Read the model definition and answer for the solid it produces. Units are mm, in the model's axes. A direction names the side the tool comes from. Give positions to 0.01 mm unless a question says otherwise; leave off trailing zeros. Write each loop counter-clockwise with the first axis right and the second up, starting at its lowest first coordinate (ties: lowest second). Pieces come first, ordered by that corner, then holes. Notation, with made-up numbers: (69.5, -26.75) -> (95.5, -26.75) arc R17 cw to (95.5, -10.75) -> close; hole circle Ø4 at (1.25, 78). An arc over 180 degrees is marked (long way). Use a Markdown table: item, result.
from build123d import *

# Parameters (mm, degrees)
SKETCH1_W           = 25.25
SKETCH1_H           = 12.5
BOSS_EXTRUDE1_DEPTH = 25.055
SKETCH2_W           = 14.5
SKETCH2_H           = 5.7
CUT_EXTRUDE1_DEPTH  = 10
BOSS_EXTRUDE2_DEPTH = 15.65
SKETCH4_R           = 4.715
BOSS_EXTRUDE3_DEPTH = 14.71
SKETCH5_R           = 2.875
SKETCH6_R           = 1.835
BOSS_EXTRUDE4_DEPTH = 10
SKETCH7_R           = 3
BOSS_EXTRUDE5_DEPTH = 5
SKETCH8_R           = 2.075
BOSS_EXTRUDE6_DEPTH = 10
FILLET1_R           = 3.67


with BuildPart() as part:
    # Sketch1 → Boss-Extrude1 (new, symmetric)
    with BuildSketch(Plane.XY):
        Rectangle(SKETCH1_W, SKETCH1_H)
    extrude(amount=BOSS_EXTRUDE1_DEPTH, both=True)

    # Sketch2 → Cut-Extrude1 (cut)
    with BuildSketch(Plane(origin=(0, 0, -25.055), x_dir=(-1, 0, 0), z_dir=(0, 0, -1))):
        with Locations((0, -1.17)):
            Rectangle(SKETCH2_W, SKETCH2_H)
    extrude(amount=-CUT_EXTRUDE1_DEPTH, mode=Mode.SUBTRACT)

    # Sketch3 → Boss-Extrude2 (add)
    with BuildSketch(Plane.XY.offset(25.055)):
        with BuildLine():
            Line((-6.42, 3.78), (-2.5, 3.78))
            ThreePointArc((-2.5, 3.78), (0.705, 0.575), (-2.5, -2.63))
            Line((-2.5, -2.63), (-6.42, -2.63))
            ThreePointArc((-6.42, -2.63), (-9.625, 0.575), (-6.42, 3.78))
        make_face()
    extrude(amount=BOSS_EXTRUDE2_DEPTH)

    # Sketch4 → Boss-Extrude3 (add)
    with BuildSketch(Plane.XY.offset(25.055)):
        with Locations(Location((5.61, -1.535, 0), (0, 0, 270))):
            Circle(SKETCH4_R)
    extrude(amount=BOSS_EXTRUDE3_DEPTH)

    # Sketch5 → section 1 of loft1
    with BuildSketch(Plane.XY.offset(59.725), mode=Mode.PRIVATE) as loft1_s1:
        with Locations((5.61, -1.535)):
            Circle(SKETCH5_R)
    # loft from a face of the part (loft1)
    loft([part.faces().sort_by_distance((5.61, -1.535, 39.765))[0], loft1_s1.sketch])

    # Sketch6 → Boss-Extrude4 (add)
    with BuildSketch(Plane.XY.offset(59.725)):
        with Locations((5.61, -1.535)):
            Circle(SKETCH6_R)
    extrude(amount=BOSS_EXTRUDE4_DEPTH)

    # Sketch7 → Boss-Extrude5 (add)
    with BuildSketch(Plane.XY.offset(40.705)):
        with Locations((-4.46, 0.575)):
            Circle(SKETCH7_R)
    extrude(amount=BOSS_EXTRUDE5_DEPTH)

    # Sketch8 → Boss-Extrude6 (add)
    with BuildSketch(Plane.XY.offset(45.705)):
        with Locations((-4.46, 0.575)):
            Circle(SKETCH8_R)
    extrude(amount=BOSS_EXTRUDE6_DEPTH)

    # Fillet1
    fillet1_edges = [part.edges().sort_by_distance(p)[0] for p in [
        (12.625, -6.25, 0),
        (-12.625, -6.25, 0),
        (-12.625, 6.25, 0),
        (12.625, 6.25, 0),
    ]]
    fillet(fillet1_edges, radius=FILLET1_R)


solid = part.part
Item 1: Straight lines are drawn through the part: line 1 along Z through (x, y) = (-8.5, -0.5) (3 decimals); line 2 along Z through (x, y) = (3.25, -0.5) (3 decimals); line 3 along Y through (x, z) = (5, 28.5). For each, find the intervals that lie inside material, in ascending order. Write a range as [from, to].
Return value:
| item | result |
|---|---|
| line 1 | [-25.055, 40.705] |
| line 2 | [-15.055, 59.725] |
| line 3 | [-6.21, 3.14] |
Item 2: A cutting plane is placed at A-A (x = -4.46). Give the vertices of the cut face in (y, z) (3 decimals), then the cut area to 3 significant figures.
Return value:
| item | result |
|---|---|
| outline | (-6.25, -25.055) -> (-4.02, -25.055) -> (-4.02, -15.055) -> (1.68, -15.055) -> (1.68, -25.055) -> (6.25, -25.055) -> (6.25, 25.055) -> (3.78, 25.055) -> (3.78, 40.705) -> (3.575, 40.705) -> (3.575, 45.705) -> (2.65, 45.705) -> (2.65, 55.705) -> (-1.5, 55.705) -> (-1.5, 45.705) -> (-2.425, 45.705) -> (-2.425, 40.705) -> (-2.63, 40.705) -> (-2.63, 25.055) -> (-6.25, 25.055) -> close |
| area | 741 mm^2 |
Item 3: Each of these flat-tipped pins is pushed along its axis until it touches: P1, Ø1.5, axis at y = 4, z = 41.5, coming from the -X side; P2, Ø2, axis at x = -4.5, z = 30.5, coming from the -Y side; P3, Ø3, axis at x = -5, z = 34, coming from the +Y side; P4, Ø3, axis at x = 2.5, y = -2, coming from the +Z side (3 decimals). Where does it stop, or does it pass through?
Return value:
| item | result |
|---|---|
| P1 | x = -5.82 |
| P2 | y = -2.63 |
| P3 | y = 3.78 |
| P4 | z = 69.725 |
Item 4: A tool of negligible diameter and unlimited length cuts with its end or side. For faces 5 (the face through (-4, 1, 55.705)), 6 (the face through (0, 1.68, -20)), 7 (the face through (4, 0, 59.725)), from which of +Z, -Z, +X, -X, +Y, -Y can it reach the whole face along a straight path? Write none if from no direction.
Return value:
| item | result |
|---|---|
| face 5 | +Z, -X, +Y, -Y |
| face 6 | -Z |
| face 7 | +Z |
Item 5: A cutting plane is placed at C-C (z = 57). Give the vertices of the cut face in (x, y) (3 decimals).
Return value:
| item | result |
|---|---|
| outline | circle Ø6.252 at (5.61, -1.535) |
Item 6: A cutting plane is placed at B-B (z = 14). Give the vertices of the cut face in (x, y) (3 decimals), then the cut area to 3 significant figures.
Return value:
| item | result |
|---|---|
| outline | (-12.625, -2.58) arc R3.67 ccw to (-8.955, -6.25) -> (8.955, -6.25) arc R3.67 ccw to (12.625, -2.58) -> (12.625, 2.58) arc R3.67 ccw to (8.955, 6.25) -> (-8.955, 6.25) arc R3.67 ccw to (-12.625, 2.58) -> close |
| area | 304 mm^2 |
Item 7: For a pull along Y with two mould halves and no side action, classify faces 1 (the face through (7.25, -1, -20)), 2 (the face through (0, 6.25, 0)), 3 (the face through (12.625, 0, 0)), 4 (the face through (-9.624, 0.505, 32.77)) as +Y half, -Y half, draft (parallel to the pull), parting line (faces both ways), or undercut.
Return value:
| item | result |
|---|---|
| face 1 | undercut |
| face 2 | +Y half |
| face 3 | draft |
| face 4 | parting line |
